Design review of the part built by this model. Coordinates are the model's own, in mm. A direction names the side the tool comes from. Give positions to 0.01 mm unless a question says otherwise; leave off trailing zeros. Order: outer loops, then holes, each group sorted by start corner. A loop starts at its lowest first (then second) coordinate and runs counter-clockwise, first axis right, second up. Notation, with made-up numbers: (31.25, -35) -> (75.25, -35) arc R28 ccw to (75.25, -12) -> close; hole circle Ø1 at (48.5, -11.75). An arc over 180 degrees is marked (long way). One line per item, written item: value.
from build123d import *

# Parameters (mm, degrees)
SKETCH_1_W          = 10
SKETCH_1_H          = 10
EXTRUDE_1_DEPTH     = 5
EXTRUDE_2_DEPTH     = 10
SKETCH_3_W          = 4.05
SKETCH_3_H          = 3.3
CUT_EXTRUDE_1_DEPTH = 1.8
SKETCH_4_W          = 4.05
SKETCH_4_H          = 1.8
CUT_EXTRUDE_2_DEPTH = 11.257801909
FILLET_1_R          = 1
EXTRUDE_3_DEPTH     = 6.65


with BuildPart() as part:
    # 草图1 → 凸台-拉伸1 (new body)
    with BuildSketch(Plane(origin=(0, 0, 0), x_dir=(1, 0, 0), z_dir=(0, 1, 0))):
        Rectangle(SKETCH_1_W, SKETCH_1_H)
    extrude(amount=EXTRUDE_1_DEPTH)

    # 草图2 → 凸台-拉伸2 (add)
    with BuildSketch(Plane(origin=(0, 0, -5), x_dir=(-1, 0, 0), z_dir=(0, 0, -1))):
        Polygon((5, 1.25), (5, 3.75), (6, 2.5), align=None)
        Polygon((-5, 1.25), (-5, 3.75), (-6, 2.5), align=None)
    extrude(amount=-EXTRUDE_2_DEPTH)

    # 草图3 → 切除-拉伸1 (cut)
    with BuildSketch(Plane(origin=(0, 5, 0), x_dir=(1, 0, 0), z_dir=(0, 1, 0))):
        Rectangle(SKETCH_3_W, SKETCH_3_H)
    extrude(amount=-CUT_EXTRUDE_1_DEPTH, mode=Mode.SUBTRACT)

    # 草图4 → 切除-拉伸2 (cut, through all)
    with BuildSketch(Plane(origin=(0, 0, 1.65), x_dir=(-1, 0, 0), z_dir=(0, 0, -1))):
        with Locations((0, 4.1)):
            Rectangle(SKETCH_4_W, SKETCH_4_H)
    extrude(amount=-CUT_EXTRUDE_2_DEPTH, mode=Mode.SUBTRACT)

    # 圆角1
    fillet_1_edges = [part.edges().sort_by_distance(p)[0] for p in [
        (0, 3.2, 5),
    ]]
    fillet(fillet_1_edges, radius=FILLET_1_R)

    # 草图5 → 凸台-拉伸3 (add)
    with BuildSketch(Plane.XY.offset(-1.65)):
        Polygon((2.025, 5), (2.025, 4.2), (1.225, 5), align=None)
        Polygon((-2.025, 4.2), (-1.225, 5), (-2.025, 5), align=None)
    extrude(amount=EXTRUDE_3_DEPTH)


solid = part.part
Item 1: Machinability: for faces 1 (the flat face through (0, 3.2, 1)), 2 (the flat face through (-5, 1, 0)), 3 (the flat face through (5, 4, 0)), 4 (the flat face through (-5, 4, 0)), which of the approach directions +Z, -Z, +X, -X, +Y, -Y give a long, thin tool a straight path to every point of the face, cutting with its end or side? Answer none if there is none.
Returned:
face 1: +Z
face 2: +Z, -Z, -X, -Y
face 3: +Z, -Z, +X, +Y
face 4: +Z, -Z, -X, +Y
Item 2: To check wall thickness, follow line 1 along X through (y, z) = (3.85, 0) (3 decimals); line 2 along Y through (x, z) = (0.25, 1); line 3 along X through (y, z) = (3.6, -1.5) (3 decimals). State the ranges of each line that lie inside material, in increasing order. Write a range as from..to.
Returned:
line 1: -5..-2.025, 2.025..5
line 2: 0..3.2
line 3: -5.12..-2.025, 2.025..5.12
Item 3: Add section C-C on z = -3.75. Give the boundary of the cut face in (x, y).
Returned:
outline: (-6, 2.5) -> (-5, 1.25) -> (-5, 0) -> (5, 0) -> (5, 1.25) -> (6, 2.5) -> (5, 3.75) -> (5, 5) -> (-5, 5) -> (-5, 3.75) -> close
Item 4: Clearance check with flat-ended pins moving along their axes: P1, Ø1, axis at y = 3.5, z = 2.5, coming from the -X side; P2, Ø1.4, axis at y = 0.5, z = 1, coming from the +X side; P3, Ø4.5, axis at x = -1, z = 2, coming from the +Y side; P4, Ø1.4, axis at y = 0.5, z = 2.5, coming from the -X side. State where each tip first meets the part, or that it passes through.
Returned:
P1: x = -5.6
P2: x = 5
P3: y = 5
P4: x = -5
Item 5: Add section B-B on x = -0.5. Give the boundary of the cut face in (y, z).
Returned:
outline: (0, -5) -> (5, -5) -> (5, -1.65) -> (3.2, -1.65) -> (3.2, 4) arc R1 ccw to (2.2, 5) -> (0, 5) -> close
Item 6: Add section D-D on z = 3.25. Give the boundary of the cut face in (x, y) (3 decimals).
Returned:
outline: (-6, 2.5) -> (-5, 1.25) -> (-5, 0) -> (5, 0) -> (5, 1.25) -> (6, 2.5) -> (5, 3.75) -> (5, 5) -> (1.225, 5) -> (2.025, 4.2) -> (2.025, 3.2) -> (-2.025, 3.2) -> (-2.025, 4.2) -> (-1.225, 5) -> (-5, 5) -> (-5, 3.75) -> close
Item 7: Add section A-A on y = 3.5. Give the boundary of the cut face in (x, z) (3 decimals).
Returned:
outline: (-5.2, -5) -> (5.2, -5) -> (5.2, 5) -> (2.025, 5) -> (2.025, -1.65) -> (-2.025, -1.65) -> (-2.025, 5) -> (-5.2, 5) -> close
